Print and shaded views of the part. All mm, measured from the part's lowest x, y and z. Coordinates: 2 decimals unless noted, no trailing zeros. Order: outer loops, then holes, each group sorted by start corner. A loop starts at its lowest first (then second) coordinate and runs counter-clockwise, first axis right, second up. Notation, with made-up numbers: (70, -23) - (123, -23) arc R19 ccw to (123, -7) - close; hole circle Ø8 at (-20, 26.25). An arc over 180 degrees is marked (long way). Write each question's results on one line, items separated by ' | '.
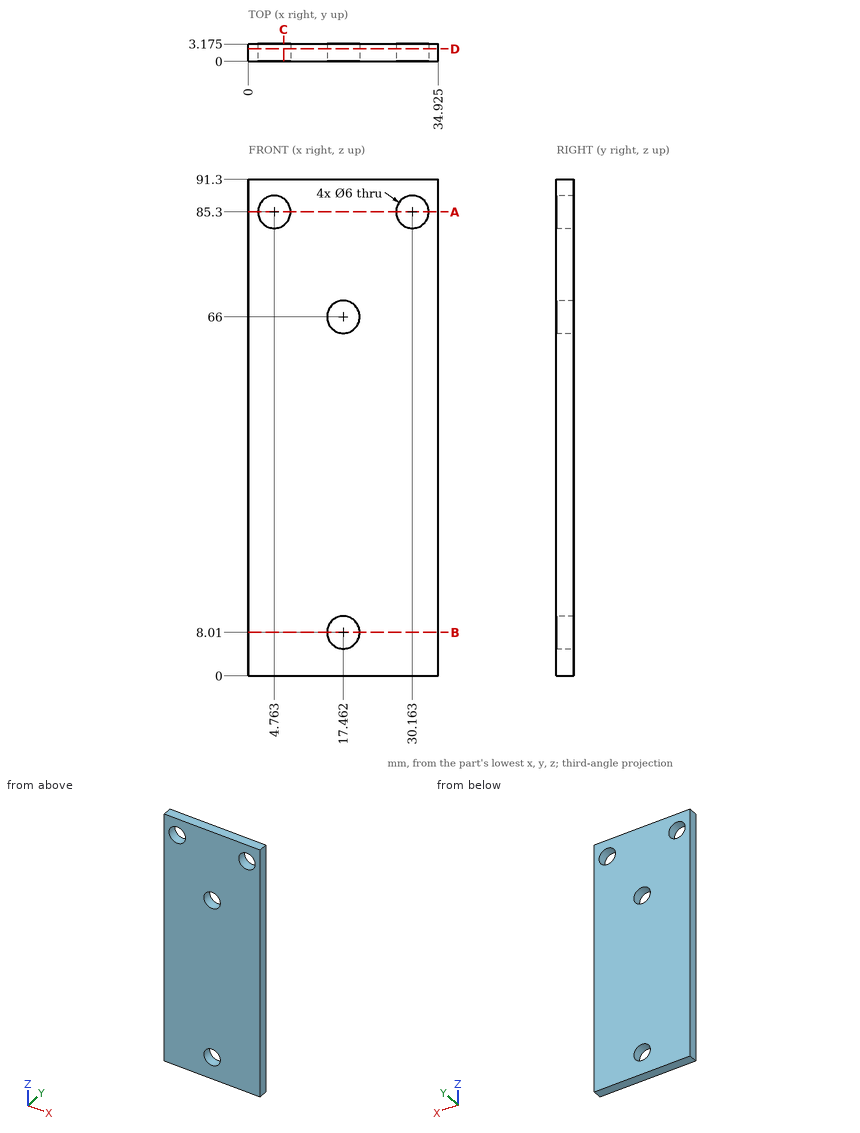
1. Band-saw the part on C-C on x = 6.5. Give the cut face in (y, z) (1 decimal).
Solved:
outline: (0, 0) - (3.2, 0) - (3.2, 82.9) - (0, 82.9) - close; (0, 87.7) - (3.2, 87.7) - (3.2, 91.3) - (0, 91.3) - close
2. Band-saw the part on D-D on y = 2.3. Give the cut face in (x, z) (1 decimal).
Solved:
outline: (0, 0) - (34.9, 0) - (34.9, 91.3) - (0, 91.3) - close; hole circle Ø6 at (4.8, 85.3); hole circle Ø6 at (17.5, 8); hole circle Ø6 at (17.5, 66); hole circle Ø6 at (30.2, 85.3)
3. Band-saw the part on B-B on z = 8.01. Give the cut face in (x, y) (1 decimal).
Solved:
outline: (0, 0) - (14.5, 0) - (14.5, 3.2) - (0, 3.2) - close; (20.5, 0) - (34.9, 0) - (34.9, 3.2) - (20.5, 3.2) - close
4. Probe line 1 (X direction, y = 1.3, z = 85.3) (1 decimal); line 2 (X direction, y = 1, z = 8.01) (1 decimal); line 3 (Z direction, x = 4.5, y = 2.9). List the from-to ranges inside material, lowest first.
Solved:
line 1: x = 0 to 1.8, 7.8 to 27.2, 33.2 to 34.9 | line 2: x = 0 to 14.5, 20.5 to 34.9 | line 3: z = 0 to 82.31, 88.29 to 91.3
5. Band-saw the part on A-A on z = 85.3. Give the cut face in (x, y) (1 decimal).
Solved:
outline: (0, 0) - (1.8, 0) - (1.8, 3.2) - (0, 3.2) - close; (7.8, 0) - (27.2, 0) - (27.2, 3.2) - (7.8, 3.2) - close; (33.2, 0) - (34.9, 0) - (34.9, 3.2) - (33.2, 3.2) - close
